The model under review builds one solid part; all positions refer to its coordinate system, in mm. A direction names the side the tool comes from. Coordinates: 2 decimals unless noted, no trailing zeros. Write each loop counter-clockwise with the first axis right and the second up, starting at its lowest first coordinate (ties: lowest second). Pieces come first, ordered by that corner, then holes. Notation, with made-up numbers: (27, 7.5) - (78, 7.5) arc R19 ccw to (78, 14.5) - close; hole circle Ø3 at (18, -39). An arc over 180 degrees is marked (long way). Put each result on its own line as item: value.
from build123d import *

# Parameters (mm, degrees)
SKETCH3_W           = 315
SKETCH3_H           = 170
BOSS_EXTRUDE1_DEPTH = 3
SKETCH5_W           = 6
SKETCH5_H           = 6
SKETCH5_W_2         = 10
SKETCH5_H_2         = 10
SKETCH5_W_3         = 10.000000001
BOSS_EXTRUDE2_DEPTH = 2
SKETCH6_R           = 2.65
CUT_EXTRUDE1_DEPTH  = 3.2
SKETCH7_R           = 1.6
CUT_EXTRUDE2_DEPTH  = 354.341194881
SKETCH8_R           = 2.8
BOSS_EXTRUDE3_DEPTH = 10
CHAMFER1_SIZE       = 1
SKETCH9_W           = 315
SKETCH9_H           = 3
BOSS_EXTRUDE4_DEPTH = 28
SKETCH10_W          = 315
SKETCH10_H          = 10
BOSS_EXTRUDE5_DEPTH = 3
CHAMFER2_SIZE       = 7
CUT_EXTRUDE3_DEPTH  = 22
SKETCH12_W          = 14.5
SKETCH12_H          = 3.389246664
BOSS_EXTRUDE6_DEPTH = 18
SKETCH13_R          = 1.6
CUT_EXTRUDE4_DEPTH  = 3.389246664
SKETCH14_W          = 14
SKETCH14_H          = 8
CUT_EXTRUDE5_DEPTH  = 2


with BuildPart() as part:
    # Sketch3 → Boss-Extrude1 (new body)
    with BuildSketch(Plane(origin=(0, 0, 0), x_dir=(1, 0, 0), z_dir=(0, 1, 0))):
        with Locations((157.5, 75)):
            Rectangle(SKETCH3_W, SKETCH3_H)
    extrude(amount=BOSS_EXTRUDE1_DEPTH)

    # Sketch5 → Boss-Extrude2 (add)
    with BuildSketch(Plane(origin=(0, 3, 0), x_dir=(1, 0, 0), z_dir=(0, 1, 0))):
        with Locations((3, 147)):
            Rectangle(SKETCH5_W, SKETCH5_H)
        with Locations((3, 3)):
            Rectangle(SKETCH5_W, SKETCH5_H)
        with Locations((6.687473524, 61.969040414)):
            Rectangle(SKETCH5_W_2, SKETCH5_H_2)
        with Locations((54.760126517, 76.409830141)):
            Rectangle(SKETCH5_W_3, SKETCH5_H_2)
        with Locations((56.888706053, 33.647880775)):
            Rectangle(SKETCH5_W_2, SKETCH5_H_2)
        with Locations((105.328256476, 112.374037416)):
            Rectangle(SKETCH5_W_2, SKETCH5_H_2)
        with Locations((108.244116471, 58.640246108)):
            Rectangle(SKETCH5_W_2, SKETCH5_H_2)
        with Locations((148.295993654, 86.70517668)):
            Rectangle(SKETCH5_W_2, SKETCH5_H_2)
        with Locations((148.852724672, 22.047319758)):
            Rectangle(SKETCH5_W_2, SKETCH5_H_2)
        with Locations((149.108148483, 8.440789408)):
            Rectangle(SKETCH5_W, SKETCH5_H)
        with Locations((196.731592235, 58.70008969)):
            Rectangle(SKETCH5_W_2, SKETCH5_H_2)
        with Locations((206.112878642, 107.13858398)):
            Rectangle(SKETCH5_W_2, SKETCH5_H_2)
        with Locations((160.584813344, 116.030051039)):
            Rectangle(SKETCH5_W, SKETCH5_H)
        with Locations((260.487872979, 11.781843085)):
            Rectangle(SKETCH5_W_2, SKETCH5_H_2)
        with Locations((290.058812632, 43.173516523)):
            Rectangle(SKETCH5_W_3, SKETCH5_H_2)
        with Locations((312, 147)):
            Rectangle(SKETCH5_W, SKETCH5_H)
        with Locations((312, 3)):
            Rectangle(SKETCH5_W, SKETCH5_H)
    extrude(amount=BOSS_EXTRUDE2_DEPTH)

    # Sketch6 → Cut-Extrude1 (cut)
    with BuildSketch(Plane(origin=(0, 0, 0), x_dir=(1, 0, 0), z_dir=(0, 1, 0))):
        with Locations(Location((3, 147, 0), (0, 0, 270))):
            Circle(SKETCH6_R)
        with Locations(Location((3, 3, 0), (0, 0, 270))):
            Circle(SKETCH6_R)
        with Locations(Location((149.108148483, 8.440789408, 0), (0, 0, 270))):
            Circle(SKETCH6_R)
        with Locations(Location((160.584813344, 116.030051039, 0), (0, 0, 270))):
            Circle(SKETCH6_R)
        with Locations(Location((312, 3, 0), (0, 0, 270))):
            Circle(SKETCH6_R)
        with Locations(Location((312, 147, 0), (0, 0, 270))):
            Circle(SKETCH6_R)
    extrude(amount=CUT_EXTRUDE1_DEPTH, mode=Mode.SUBTRACT)

    # Sketch7 → Cut-Extrude2 (cut, through all)
    with BuildSketch(Plane(origin=(0, 0, 0), x_dir=(1, 0, 0), z_dir=(0, 1, 0))):
        with Locations(Location((3, 147, 0), (0, 0, 270))):
            Circle(SKETCH7_R)
        with Locations(Location((312, 147, 0), (0, 0, 270))):
            Circle(SKETCH7_R)
        with Locations(Location((312, 3, 0), (0, 0, 270))):
            Circle(SKETCH7_R)
        with Locations(Location((149.108148483, 8.440789408, 0), (0, 0, 270))):
            Circle(SKETCH7_R)
        with Locations(Location((160.584813344, 116.030051039, 0), (0, 0, 270))):
            Circle(SKETCH7_R)
        with Locations(Location((3, 3, 0), (0, 0, 270))):
            Circle(SKETCH7_R)
    extrude(amount=CUT_EXTRUDE2_DEPTH, mode=Mode.SUBTRACT)

    # Sketch8 → Boss-Extrude3 (add)
    with BuildSketch(Plane(origin=(0, 0, 0), x_dir=(1, 0, 0), z_dir=(0, 1, 0))):
        with Locations(Location((6.687473524, 61.969040414, 0), (0, 0, 270))):
            Circle(SKETCH8_R)
        with Locations(Location((54.760126516, 76.409830141, 0), (0, 0, 270))):
            Circle(SKETCH8_R)
        with Locations(Location((56.888706053, 33.647880775, 0), (0, 0, 270))):
            Circle(SKETCH8_R)
        with Locations(Location((108.244116471, 58.640246108, 0), (0, 0, 270))):
            Circle(SKETCH8_R)
        with Locations(Location((105.328256476, 112.374037416, 0), (0, 0, 270))):
            Circle(SKETCH8_R)
        with Locations(Location((148.295993654, 86.70517668, 0), (0, 0, 270))):
            Circle(SKETCH8_R)
        with Locations(Location((206.112878642, 107.13858398, 0), (0, 0, 270))):
            Circle(SKETCH8_R)
        with Locations(Location((196.731592235, 58.70008969, 0), (0, 0, 270))):
            Circle(SKETCH8_R)
        with Locations(Location((148.852724672, 22.047319758, 0), (0, 0, 270))):
            Circle(SKETCH8_R)
        with Locations(Location((260.487872979, 11.781843085, 0), (0, 0, 270))):
            Circle(SKETCH8_R)
        with Locations(Location((290.058812632, 43.173516523, 0), (0, 0, 270))):
            Circle(SKETCH8_R)
    extrude(amount=BOSS_EXTRUDE3_DEPTH)

    # Chamfer1
    chamfer1_edges = [part.edges().sort_by_distance(p)[0] for p in [
        (6.687473524, 10, -64.769040414),
        (54.760126516, 10, -79.209830141),
        (56.888706053, 10, -36.447880775),
        (108.244116471, 10, -61.440246108),
        (105.328256476, 10, -115.174037416),
        (148.295993654, 10, -89.50517668),
        (206.112878642, 10, -109.93858398),
        (196.731592235, 10, -61.50008969),
        (148.852724672, 10, -24.847319758),
        (260.487872979, 10, -14.581843085),
        (290.058812632, 10, -45.973516523),
    ]]
    chamfer(chamfer1_edges, length=CHAMFER1_SIZE)

    # Sketch9 → Boss-Extrude4 (add)
    with BuildSketch(Plane(origin=(0, 0, 0), x_dir=(1, 0, 0), z_dir=(0, 1, 0))):
        with Locations((157.5, 158.5)):
            Rectangle(SKETCH9_W, SKETCH9_H)
        with Locations((157.5, -8.5)):
            Rectangle(SKETCH9_W, SKETCH9_H)
    extrude(amount=BOSS_EXTRUDE4_DEPTH)

    # Sketch10 → Boss-Extrude5 (add)
    with BuildSketch(Plane(origin=(0, 28, 0), x_dir=(1, 0, 0), z_dir=(0, 1, 0))):
        with Locations((157.5, 155)):
            Rectangle(SKETCH10_W, SKETCH10_H)
        with Locations((157.5, -5)):
            Rectangle(SKETCH10_W, SKETCH10_H)
    extrude(amount=-BOSS_EXTRUDE5_DEPTH)

    # Chamfer2
    chamfer2_edges = [part.edges().sort_by_distance(p)[0] for p in [
        (157.5, 25, 7),
        (157.5, 25, -157),
    ]]
    chamfer(chamfer2_edges, length=CHAMFER2_SIZE - 0.0001)  # a hair under: the kernel refuses the full size
    chamfer2_2_edges = [part.edges().sort_by_distance(p)[0] for p in [
        (157.5, 28, 10),
        (157.5, 28, -160),
    ]]
    chamfer(chamfer2_2_edges, length=CHAMFER2_SIZE)

    # Sketch11 → Cut-Extrude3 (cut)
    with BuildSketch(Plane(origin=(0, 0, -160), x_dir=(-1, 0, 0), z_dir=(0, 0, -1))):
        Polygon((-277.845030897, 9.289246664), (-285.445030897, 9.289246664), (-285.445030897, 7.989246664), (-284.745030897, 7.289246664), (-278.545030897, 7.289246664), (-277.845030897, 7.989246664), align=None)
    extrude(amount=-CUT_EXTRUDE3_DEPTH, mode=Mode.SUBTRACT)

    # Sketch12 → Boss-Extrude6 (add)
    with BuildSketch(Plane(origin=(0, 0, -160), x_dir=(-1, 0, 0), z_dir=(0, 0, -1))):
        with Locations((-281.645030897, 4.694623332)):
            Rectangle(SKETCH12_W, SKETCH12_H)
    extrude(amount=-BOSS_EXTRUDE6_DEPTH)

    # Sketch13 → Cut-Extrude4 (cut)
    with BuildSketch(Plane(origin=(0, 6.389246664, 0), x_dir=(1, 0, 0), z_dir=(0, 1, 0))):
        with Locations(Location((277.395030897, 148.487326261, 0), (0, 0, 180))):
            Circle(SKETCH13_R)
        with Locations(Location((285.895030897, 148.487326261, 0), (0, 0, 180))):
            Circle(SKETCH13_R)
    extrude(amount=-CUT_EXTRUDE4_DEPTH, mode=Mode.SUBTRACT)

    # Sketch14 → Cut-Extrude5 (cut)
    with BuildSketch(Plane(origin=(0, 0, -160), x_dir=(-1, 0, 0), z_dir=(0, 0, -1))):
        with Locations((-281.645030897, 8.289246664)):
            Rectangle(SKETCH14_W, SKETCH14_H)
    extrude(amount=-CUT_EXTRUDE5_DEPTH, mode=Mode.SUBTRACT)


solid = part.part
1. To check wall thickness, follow probe 1 along X at (y, z) = (2.45, -3); probe 2 along Z at (x, y) = (108.5, 6); probe 3 along Z at (x, y) = (202.5, 3.25). State the ranges of each line that lie inside material, in increasing order.
Determined:
probe 1: x = 0 to 0.35, 5.65 to 309.35, 314.65 to 315
probe 2: z = -160 to -157, -61.43 to -55.85, 7 to 10
probe 3: z = -160 to -157, -112.14 to -102.14, 7 to 10
2. Machinability: for faces 4 (the flat face through (0, 2, -62)), 5 (the flat face through (310.6, 5, -4.4)), 6 (the flat face through (107.5, 5, -110.2)), which of the approach directions +Z, -Z, +X, -X, +Y, -Y give a long, thin tool a straight path to every point of the face, cutting with its end or side? Answer none if there is none.
Determined:
face 4: +Z, -Z, -X, +Y, -Y
face 5: +X, -X, +Y
face 6: +Y
3. For pin 1 Ø12 at (y, z) = (13, -104.5) entering from -X; pin 2 Ø1.8 at (x, z) = (261, -12) entering from +Y; pin 3 Ø0.6 at (y, z) = (4, -117) entering from +X; pin 4 Ø1.9 at (x, z) = (3, -3) entering from +Y, all flat-tipped, find the tip position at first contact; note any pin that passes through.
Determined:
pin 1: stops at x = 203.31
pin 2: stops at y = 10
pin 3: stops at x = 163.58
pin 4: passes through
4. The part is to be moulded in two halves that separate along Z. For faces 1 (the flat face through (1.6, 5, -4.4)), 2 (the flat face through (155, 24, -157)), 3 (the flat face through (315, 2, -62)), say which applies: +Z half, -Z half, draft (parallel to the pull), parting line (faces both ways), or undercut.
Determined:
face 1: undercut
face 2: -Z half
face 3: draft
5. Consider section B-B on z = -129.5. State the section outline as (x, y) points.
Determined:
outline: (0, 0) - (315, 0) - (315, 3) - (0, 3) - close
